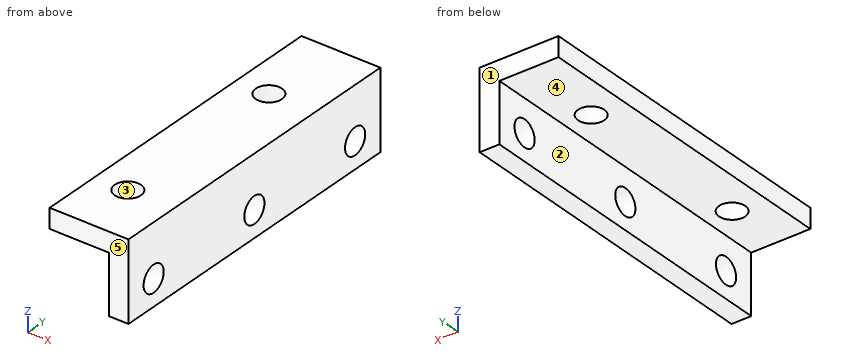
Autodesk Inventor part; units mm, degrees
ref_plane "YZ Plane" through (0, 0, 0) normal (1, 0, 0) x (0, 1, 0)
ref_plane "XZ Plane" through (0, 0, 0) normal (0, 1, 0) x (-1, 0, 0)
ref_plane "XY Plane" through (0, 0, 0) normal (0, 0, 1) x (1, 0, 0)
sketch "Skizze1" plane through (0, 0, 0) normal (0, 1, 0) x (-1, 0, 0)
  line L0 (0, 0) -> (12, 0)
  line L1 (12, 0) -> (12, -3)
  line L2 (12, -3) -> (3, -3)
  line L3 (3, -3) -> (3, -12)
  line L4 (3, -12) -> (0, -12)
  line L5 (0, -12) -> (0, 0)
  dimension "d0" = 12
  dimension "d1" = 3
  dimension "d2" = 12
  dimension "d3" = 3
extrude "Extrusion1" add sketch "Skizze1" along normal blind 50
sketch "Skizze2" plane through (-3, 0, -12) normal (-1, 0, 0) x (0, 0, 1)
  line L0 (0, 0) -> (0, 50)
  line L1 (12, 0) -> (0, 0)
  line L2 (0, 50) -> (9, 50)
  point P0 (4, 45)
  point P1 (4, 5)
  point P2 (0, 25)
  point P3 (4, 25)
  dimension "d13" = 4
  dimension "d29" = 5
  dimension "d30" = 5
  dimension "d31" = 20
hole "Bohrung1" at (-3, 45, -8) at (-3, 5, -8) at (-3, 25, -8) direction (1, 0, 0) diameter 4 end through all
sketch "Skizze3" plane through (-3, 0, -3) normal (0, 0, -1) x (-1, 0, 0)
  line L0 (0, 0) -> (9, 0)
  line L1 (0, 50) -> (9, 50)
  line L2 (9, 0) -> (9, 50)
  point P0 (-3, 0)
  point P1 (4, 9)
  point P2 (4, 37)
  point P3 (4.5, 0)
  point P4 (9, 25)
  dimension "d26" = 28
  dimension "d28" = 5
  dimension "d32" = 9
hole "Bohrung2" at (-7, 9, -3) at (-7, 37, -3) direction (0, 0, 1) diameter 4 end through all
properties part number "1172" material "Aluminium 6061"
Input: part model. Units: mm. Frame: model coordinates. Face numbers are marked on the shaded views. A direction names the side the tool comes from. Round coordinates to 2 decimals unless told otherwise and drop trailing zeros. Order: outer loops, then holes, each group sorted by start corner. A loop starts at its lowest first (then second) coordinate and runs counter-clockwise, first axis right, second up.
1. Mould query, pull axis Y, two halves, no side actions, for the marked faces 3, 4 and 5. Classes: released by +Y, released by -Y, zero draft, split by the parting line, or undercut.
The answers:
face 3: undercut
face 4: zero draft
face 5: released by -Y
2. Cut plane D-D, the plane x = -2.25. Output: boundary loops of the cut face in (y, z).
The answers:
outline: (0, -12) - (50, -12) - (50, 0) - (0, 0) - close; hole circle Ø4 at (5, -8); hole circle Ø4 at (25, -8); hole circle Ø4 at (45, -8)
3. Set-up query: the marked faces 1 and 2. Return all of +Z, -Z, +X, -X, +Y, -Y with unobstructed straight access to the full face (end or side cutting, diameter ignored); none if empty.
The answers:
face 1: +Z, -Z, +X, -X, +Y
face 2: -Z, -X, +Y, -Y
4. Material intervals for line 1 (Y direction, x = -1.5, z = -8); line 2 (Y direction, x = -7, z = -2.05); line 3 (Z direction, x = -1.3, y = 45), sorted ascending.
The answers:
line 1: y = 0 to 3, 7 to 23, 27 to 43, 47 to 50
line 2: y = 0 to 7, 11 to 35, 39 to 50
line 3: z = -12 to -10, -6 to 0
5. Pin query (flat end, axial travel): P1, Ø5, axis at x = -7, y = 9, coming from the -Z side; P2, Ø5, axis at y = 5, z = -8, coming from the -X side; P3, Ø3.5, axis at x = -7, y = 37, coming from the -Z side. Return the tip coordinate at first contact, or that it passes through.
The answers:
P1: stops at z = -3
P2: stops at x = -3
P3: passes through
6. Cut plane C-C, the plane y = 25. Output: boundary loops of the cut face in (x, z).
The answers:
outline: (-12, -3) - (-3, -3) - (-3, -6) - (0, -6) - (0, 0) - (-12, 0) - close; (-3, -12) - (0, -12) - (0, -10) - (-3, -10) - close
7. Cut plane B-B, the plane x = -7. Output: boundary loops of the cut face in (y, z), then the cut area to 3 significant figures.
The answers:
outline: (0, -3) - (7, -3) - (7, 0) - (0, 0) - close; (11, -3) - (35, -3) - (35, 0) - (11, 0) - close; (39, -3) - (50, -3) - (50, 0) - (39, 0) - close
area: 126 mm2
8. Cut plane A-A, the plane z = -8. Output: boundary loops of the cut face in (x, y).
The answers:
outline: (-3, 0) - (0, 0) - (0, 3) - (-3, 3) - close; (-3, 7) - (0, 7) - (0, 23) - (-3, 23) - close; (-3, 27) - (0, 27) - (0, 43) - (-3, 43) - close; (-3, 47) - (0, 47) - (0, 50) - (-3, 50) - close
